Geometry: final body of the model. Coordinates: model frame, mm. A direction names the side the tool comes from. Coordinates: 2 decimals unless noted, no trailing zeros. Write each loop counter-clockwise with the first axis right and the second up, starting at its lowest first coordinate (ties: lowest second). Pieces come first, ordered by that corner, then holes. Notation, with made-up numbers: (49.25, -24.5) - (97.25, -24.5) arc R23 ccw to (97.25, -10.5) - close; hole circle Ø9 at (52.5, 5). An arc over 180 degrees is marked (long way). Put each result on its own line as item: value.
Autodesk Fusion 360 part; units mm, degrees
sketch "Esquisse1" plane through (0, 0, 0) normal (0, 0, 1) x (1, 0, 0)
  line L0 (9.4, 40) -> (70, 40)
  line L1 (70, 40) -> (70, 23.65)
  line L2 (70, 23.65) -> (9.4, 23.65)
  line L3 (9.4, 23.65) -> (9.4, 40)
  dimension "d1" = 60.6
  dimension "d2" = 16.35
extrude "Extrusion1" add sketch "Esquisse1" along normal blind 3
sketch "Esquisse2" plane through (0, 0, 0) normal (0, 0, -1) x (1, 0, 0)
  line L0 (70, -23.65) -> (9.4, -23.65)
  line L1 (9.4, -23.65) -> (9.4, -40)
  line L2 (9.4, -40) -> (70, -40)
  line L3 (70, -40) -> (70, -23.65)
  line L4 (17.1, -25.55) -> (22.3, -25.55)
  line L5 (22.3, -25.55) -> (22.3, -27.75)
  line L6 (22.3, -27.75) -> (17.1, -27.75)
  line L7 (17.1, -27.75) -> (17.1, -25.55)
  line L8 (19.7, -25.55) -> (19.7, -27.75) construction
  line L9 (39.7, -23.65) -> (39.7, -40) construction
  line L10 (57.1, -25.55) -> (57.1, -27.75)
  line L11 (62.3, -25.55) -> (57.1, -25.55)
  line L12 (62.3, -27.75) -> (62.3, -25.55)
  line L13 (57.1, -27.75) -> (62.3, -27.75)
  line L14 (9.4, -31.825) -> (70, -31.825) construction
  line L15 (17.1, -38.1) -> (22.3, -38.1)
  line L16 (22.3, -38.1) -> (22.3, -35.9)
  line L17 (22.3, -35.9) -> (17.1, -35.9)
  line L18 (17.1, -35.9) -> (17.1, -38.1)
  line L19 (62.3, -38.1) -> (57.1, -38.1)
  line L20 (62.3, -35.9) -> (62.3, -38.1)
  line L21 (57.1, -35.9) -> (62.3, -35.9)
  line L22 (57.1, -38.1) -> (57.1, -35.9)
  dimension "d5" = 20
  dimension "d12" = 5.2
  dimension "d13" = 2.2
  dimension "d14" = 1.9
extrude "Extrusion2" cut sketch "Esquisse2" against normal blind 2 contours L4 L5 L6 L7 | L10 L11 L12 L13 | L15 L16 L17 L18 | L19 L20 L21 L22
sketch "Esquisse3" plane through (0, 0, 3) normal (0, 0, 1) x (-1, 0, 0)
  line L0 (-9.4, -23.65) -> (-70, -23.65)
  line L1 (-70, -23.65) -> (-70, -40)
  line L2 (-70, -40) -> (-9.4, -40)
  line L3 (-9.4, -40) -> (-9.4, -23.65)
  line L4 (-26.95, -39.525) -> (-52.45, -39.525)
  line L5 (-52.45, -39.525) -> (-52.45, -24.125)
  line L6 (-52.45, -24.125) -> (-26.95, -24.125)
  line L7 (-26.95, -24.125) -> (-26.95, -39.525)
  line L8 (-9.4, -31.825) -> (-70, -31.825) construction
  line L9 (-39.7, -40) -> (-39.7, -23.65) construction
  dimension "d8" = 25.5
  dimension "d9" = 15.4
extrude "Extrusion3" cut sketch "Esquisse3" against normal blind 2 contours L4 L5 L6 L7
sketch "Esquisse4" plane through (0, 0, 1) normal (0, 0, 1) x (-1, 0, 0)
  line L0 (-26.95, -24.125) -> (-52.45, -24.125)
  line L1 (-52.45, -24.125) -> (-52.45, -39.525)
  line L2 (-52.45, -39.525) -> (-26.95, -39.525)
  line L3 (-26.95, -39.525) -> (-26.95, -24.125)
  line L4 (-26.95, -24.125) -> (-29.95, -24.125)
  line L5 (-29.95, -24.125) -> (-29.95, -39.525)
  line L6 (-29.95, -39.525) -> (-26.95, -39.525)
  line L7 (-26.95, -39.525) -> (-26.95, -24.125)
  dimension "d15" = 3
extrude "Extrusion4" cut sketch "Esquisse4" against normal blind 3 contours L0 L2 L3 L4 L5 L6 L7
sketch "Esquisse5" plane through (0, 40, 0) normal (0, 1, 0) x (-1, 0, 0)
  line L0 (-70, 0) -> (-9.4, 0)
  line L1 (-9.4, 0) -> (-9.4, 3)
  line L2 (-9.4, 3) -> (-70, 3)
  line L3 (-70, 3) -> (-70, 0)
  line L4 (-39.7, 3) -> (-39.7, 0) construction
  line L5 (-47.2, 3) -> (-32.2, 3)
  line L6 (-32.2, 3) -> (-32.2, 1)
  line L7 (-32.2, 1) -> (-47.2, 1)
  line L8 (-47.2, 1) -> (-47.2, 3)
  dimension "d18" = 15
  dimension "d19" = 2
extrude "Extrusion5" cut sketch "Esquisse5" against normal blind 21 contours L2 L5 L6 L7 L8
sketch "Esquisse6" plane through (0, 0, 3) normal (0, 0, 1) x (-1, 0, 0)
  line L0 (-47.2, -24.125) -> (-47.2, -23.65)
  line L1 (-47.2, -23.65) -> (-70, -23.65)
  line L2 (-70, -23.65) -> (-70, -40)
  line L3 (-70, -40) -> (-47.2, -40)
  line L4 (-47.2, -40) -> (-47.2, -39.525)
  line L5 (-47.2, -39.525) -> (-52.45, -39.525)
  line L6 (-52.45, -39.525) -> (-52.45, -24.125)
  line L7 (-52.45, -24.125) -> (-47.2, -24.125)
  line L8 (-70, -40) -> (-67.5, -40)
  line L9 (-67.5, -40) -> (-67.5, -23.65)
  line L10 (-67.5, -23.65) -> (-70, -23.65)
  line L11 (-70, -23.65) -> (-70, -40)
  line L12 (-39.7, -39) -> (-39.7, -18) construction
  line L13 (-9.4, -23.65) -> (-9.4, -40)
  line L14 (-11.9, -23.65) -> (-9.4, -23.65)
  line L15 (-11.9, -40) -> (-11.9, -23.65)
  line L16 (-9.4, -40) -> (-11.9, -40)
  dimension "d22" = 2.5
  dimension "d23" = 30.3
extrude "Extrusion6" cut sketch "Esquisse6" against normal blind 2 contours L1 L2 L3 L8 L9 L10 L11 | L13 L14 L15 L16
1. Set-up query: faces 4 (the flat face through (26.95, 32, 2)), 5 (the flat face through (62.3, 27, 1)), 6 (the flat face through (59, 32, 3)), 7 (the flat face through (50, 24.125, 2)), 8 (the flat face through (39, 32, 0)). Return all of +Z, -Z, +X, -X, +Y, -Y with unobstructed straight access to the full face (end or side cutting, diameter ignored); none if empty.
Answer below:
face 4: +Z, -Z
face 5: -Z
face 6: +Z, +X, -X, +Y, -Y
face 7: +Z
face 8: -Z, +X, -X, +Y, -Y
2. Ray query, probe 1 along X at (y, z) = (38, 0.7); probe 2 along Y at (x, z) = (61, 0.8); probe 3 along X at (y, z) = (35, 2.25). Return the intervals inside material, ascending. Write a range as from..to.
Answer below:
probe 1: x = 9.4..17.1, 22.3..26.95, 29.95..57.1, 62.3..70
probe 2: y = 23.65..25.55, 27.75..35.9, 38.1..40
probe 3: x = 11.9..26.95, 52.45..67.5
3. Section query C-C (y = 38.75). Return loops of the section in (x, z), then the cut area to 3 significant figures.
Answer below:
outline: (9.4, 0) - (26.95, 0) - (26.95, 3) - (11.9, 3) - (11.9, 1) - (9.4, 1) - close; (29.95, 0) - (70, 0) - (70, 1) - (67.5, 1) - (67.5, 3) - (52.45, 3) - (52.45, 1) - (29.95, 1) - close
area: 118 mm²
4. Pin query (flat end, axial travel): pin 1 Ø0.7 at (x, y) = (60, 37) entering from -Z; pin 2 Ø6 at (x, y) = (49, 30) entering from +Z; pin 3 Ø1.5 at (y, z) = (25.5, 2) entering from -X. Return the tip coordinate at first contact, or that it passes through.
Answer below:
pin 1: stops at z = 2
pin 2: stops at z = 1
pin 3: stops at x = 11.9
5. Section query B-B (x = 27.5). Return loops of the section in (y, z) (3 decimals).
Answer below:
outline: (23.65, 0) - (24.125, 0) - (24.125, 3) - (23.65, 3) - close; (39.525, 0) - (40, 0) - (40, 3) - (39.525, 3) - close
6. Section query A-A (z = 2.5). Return loops of the section in (x, y) (3 decimals).
Answer below:
outline: (11.9, 23.65) - (32.2, 23.65) - (32.2, 24.125) - (26.95, 24.125) - (26.95, 39.525) - (32.2, 39.525) - (32.2, 40) - (11.9, 40) - close; (47.2, 23.65) - (67.5, 23.65) - (67.5, 40) - (47.2, 40) - (47.2, 39.525) - (52.45, 39.525) - (52.45, 24.125) - (47.2, 24.125) - close
7. Section query D-D (x = 49). Return loops of the section in (y, z) (3 decimals), then the cut area to 4 significant figures.
Answer below:
outline: (23.65, 0) - (40, 0) - (40, 3) - (39.525, 3) - (39.525, 1) - (24.125, 1) - (24.125, 3) - (23.65, 3) - close
area: 18.25 mm²
8. Mould query, pull axis Y, two halves, no side actions, for faces 1 (the flat face through (29.95, 31.7, 0.5)), 2 (the flat face through (39.3, 40, 0.8)), 3 (the flat face through (11.9, 32, 2)). Classes: +Y half, -Y half, draft (parallel to the pull), parting line (faces both ways), or undercut.
Answer below:
face 1: undercut
face 2: +Y half
face 3: draft
